```python
from build123d import *

# Parameters (mm, degrees)
F0_R         = 0.875
F1_DEPTH     = 12
F2_R         = 1.75
F3_DEPTH     = 4.001
F4_DEPTH     = 2
F5_T4_DEPTH  = 12
F5_T10_DEPTH = 12
F5_T16_DEPTH = 12
F5_T23_DEPTH = 12
F5_T29_DEPTH = 12
F5_T35_DEPTH = 12
F5_T41_DEPTH = 12
F5_T47_DEPTH = 12
F5_T54_DEPTH = 12
F5_T60_DEPTH = 12
F5_T63_DEPTH = 14.2867319519
F5_T65_DEPTH = 22.2867319519
F6_R         = 1


# Not quite as in the source:
# - a fillet or chamfer that OpenCascade refuses, or shapes differently, is made with other operations: its cross-section is extruded or revolved along the edge and cut away or added


with BuildPart() as f1:
    # F0 (on Top) → F1 (new body)
    with BuildSketch(Plane.XY):
        Polygon((16.5, -5.25), (11.625, -5.25), (-11.625, -5.25), (-16.5, -5.25), (-16.5, -7.25), (16.5, -7.25), align=None)
        Polygon((-11.625, -5.25), (-11.625, 7.25), (-16.5, 7.25), (-16.5, -3.25), (-16.5, -5.25), align=None)
        with Locations((-13.5, 1)):
            Circle(F0_R, mode=Mode.SUBTRACT)
        Polygon((16.5, -3.25), (16.5, 7.25), (11.625, 7.25), (11.625, -5.25), (16.5, -5.25), align=None)
        with Locations((13.5, 1)):
            Circle(F0_R, mode=Mode.SUBTRACT)
        Polygon((25.5, -3.25), (16.5, -3.25), (16.5, -5.25), (16.5, -7.25), (25.5, -7.25), align=None)
        Polygon((-16.5, -5.25), (-16.5, -3.25), (-25.5, -3.25), (-25.5, -7.25), (-16.5, -7.25), align=None)
    extrude(amount=F1_DEPTH)

    # F2 (on face) → F3 (cut, through all)
    with BuildSketch(Plane(origin=(0, -3.25, 0), x_dir=(-1, 0, 0), z_dir=(0, 1, 0))):
        with Locations((-21, 6)):
            Circle(F2_R)
        with Locations((21, 6)):
            Circle(F2_R)
    extrude(amount=-F3_DEPTH, mode=Mode.SUBTRACT)

    # F2 (on face) → F4 (cut)
    with BuildSketch(Plane(origin=(0, -3.25, 0), x_dir=(-1, 0, 0), z_dir=(0, 1, 0))):
        Polygon((-18.25, 4.4122867597), (-18.25, 7.5877132403), (-21, 9.1754264805), (-23.75, 7.5877132403), (-23.75, 4.4122867597), (-21, 2.8245735195), align=None)
        with Locations((-21, 6)):
            Circle(F2_R, mode=Mode.SUBTRACT)
        Polygon((21, 9.1754264805), (18.25, 7.5877132403), (18.25, 4.4122867597), (21, 2.8245735195), (23.75, 4.4122867597), (23.75, 7.5877132403), align=None)
        with Locations((21, 6)):
            Circle(F2_R, mode=Mode.SUBTRACT)
    extrude(amount=-F4_DEPTH, mode=Mode.SUBTRACT)

    # F5: chamfer of 2 on 8 edges, made by hand


with BuildPart() as f5_tool2:
    # F5_s3 → F5_t4 (new body)
    with BuildSketch(Plane.XY):
        Polygon((18.5, -3.25), (16.5, -1.25), (16.5, -3.25), align=None)
    extrude(amount=F5_T4_DEPTH)

    split(bisect_by=Plane.YZ.offset(18.25), keep=Keep.TOP)

    split(bisect_by=Plane(origin=(6.4730762114, 0, 11.2116968793), x_dir=(0, 1, 0), z_dir=(-0.5, 0, -0.8660254038)), keep=Keep.TOP)


with BuildPart() as f1_1:
    add(f1.part)

    # F5_t1: union F5_tool2
    add(f5_tool2.part)


with BuildPart() as f5_tool8:
    # F5_s9 → F5_t10 (new body)
    with BuildSketch(Plane.XY):
        Polygon((18.5, -3.25), (16.5, -1.25), (16.5, -3.25), align=None)
    extrude(amount=F5_T10_DEPTH)

    split(bisect_by=Plane.YZ.offset(18.25), keep=Keep.BOTTOM)

    split(bisect_by=Plane(origin=(6.4730762114, 0, 11.2116968793), x_dir=(0, 1, 0), z_dir=(-0.5, 0, -0.8660254038)), keep=Keep.TOP)


with BuildPart() as f1_2:
    add(f1_1.part)

    # F5_t7: union F5_tool8
    add(f5_tool8.part)


with BuildPart() as f5_tool14:
    # F5_s15 → F5_t16 (new body)
    with BuildSketch(Plane.XY):
        Polygon((18.5, -3.25), (16.5, -1.25), (16.5, -3.25), align=None)
    extrude(amount=F5_T16_DEPTH)

    split(bisect_by=Plane(origin=(1.2769237886, 0, -2.2116968793), x_dir=(0, 1, 0), z_dir=(0.5, 0, -0.8660254038)), keep=Keep.TOP)

    split(bisect_by=Plane.YZ.offset(18.25), keep=Keep.BOTTOM)

    split(bisect_by=Plane(origin=(6.4730762114, 0, 11.2116968793), x_dir=(0, 1, 0), z_dir=(0.5, 0, 0.8660254038)), keep=Keep.TOP)


with BuildPart() as f1_3:
    add(f1_2.part)

    # F5_t13: union F5_tool14
    add(f5_tool14.part)


with BuildPart() as f5_tool21:
    # F5_s22 → F5_t23 (new body)
    with BuildSketch(Plane.XY):
        Polygon((18.5, -3.25), (16.5, -1.25), (16.5, -3.25), align=None)
    extrude(amount=F5_T23_DEPTH)

    split(bisect_by=Plane(origin=(1.2769237886, 0, -2.2116968793), x_dir=(0, 1, 0), z_dir=(-0.5, 0, 0.8660254038)), keep=Keep.TOP)

    split(bisect_by=Plane.YZ.offset(18.25), keep=Keep.TOP)


with BuildPart() as f1_4:
    add(f1_3.part)

    # F5_t20: union F5_tool21
    add(f5_tool21.part)


with BuildPart() as f5_tool27:
    # F5_s28 → F5_t29 (new body)
    with BuildSketch(Plane.XY):
        Polygon((18.5, -3.25), (16.5, -1.25), (16.5, -3.25), align=None)
    extrude(amount=F5_T29_DEPTH)

    split(bisect_by=Plane(origin=(1.2769237886, 0, -2.2116968793), x_dir=(0, 1, 0), z_dir=(-0.5, 0, 0.8660254038)), keep=Keep.TOP)

    split(bisect_by=Plane.YZ.offset(18.25), keep=Keep.BOTTOM)


with BuildPart() as f1_5:
    add(f1_4.part)

    # F5_t26: union F5_tool27
    add(f5_tool27.part)


with BuildPart() as f5_tool33:
    # F5_s34 → F5_t35 (new body)
    with BuildSketch(Plane.XY):
        Polygon((-16.5, -1.25), (-18.5, -3.25), (-16.5, -3.25), align=None)
    extrude(amount=F5_T35_DEPTH)

    split(bisect_by=Plane(origin=(-6.4730762114, 0, 11.2116968793), x_dir=(0, 1, 0), z_dir=(0.5, 0, -0.8660254038)), keep=Keep.TOP)

    split(bisect_by=Plane.YZ.offset(-18.25), keep=Keep.TOP)


with BuildPart() as f1_6:
    add(f1_5.part)

    # F5_t32: union F5_tool33
    add(f5_tool33.part)


with BuildPart() as f5_tool39:
    # F5_s40 → F5_t41 (new body)
    with BuildSketch(Plane.XY):
        Polygon((-16.5, -1.25), (-18.5, -3.25), (-16.5, -3.25), align=None)
    extrude(amount=F5_T41_DEPTH)

    split(bisect_by=Plane(origin=(-6.4730762114, 0, 11.2116968793), x_dir=(0, 1, 0), z_dir=(0.5, 0, -0.8660254038)), keep=Keep.TOP)

    split(bisect_by=Plane.YZ.offset(-18.25), keep=Keep.BOTTOM)


with BuildPart() as f1_7:
    add(f1_6.part)

    # F5_t38: union F5_tool39
    add(f5_tool39.part)


with BuildPart() as f5_tool45:
    # F5_s46 → F5_t47 (new body)
    with BuildSketch(Plane.XY):
        Polygon((-16.5, -1.25), (-18.5, -3.25), (-16.5, -3.25), align=None)
    extrude(amount=F5_T47_DEPTH)

    split(bisect_by=Plane(origin=(-6.4730762114, 0, 11.2116968793), x_dir=(0, 1, 0), z_dir=(-0.5, 0, 0.8660254038)), keep=Keep.TOP)

    split(bisect_by=Plane.YZ.offset(-18.25), keep=Keep.TOP)

    split(bisect_by=Plane(origin=(-1.2769237886, 0, -2.2116968793), x_dir=(0, 1, 0), z_dir=(-0.5, 0, -0.8660254038)), keep=Keep.TOP)


with BuildPart() as f1_8:
    add(f1_7.part)

    # F5_t44: union F5_tool45
    add(f5_tool45.part)


with BuildPart() as f5_tool52:
    # F5_s53 → F5_t54 (new body)
    with BuildSketch(Plane.XY):
        Polygon((-16.5, -1.25), (-18.5, -3.25), (-16.5, -3.25), align=None)
    extrude(amount=F5_T54_DEPTH)

    split(bisect_by=Plane.YZ.offset(-18.25), keep=Keep.TOP)

    split(bisect_by=Plane(origin=(-1.2769237886, 0, -2.2116968793), x_dir=(0, 1, 0), z_dir=(0.5, 0, 0.8660254038)), keep=Keep.TOP)


with BuildPart() as f1_9:
    add(f1_8.part)

    # F5_t51: union F5_tool52
    add(f5_tool52.part)


with BuildPart() as f5_tool58:
    # F5_s59 → F5_t60 (new body)
    with BuildSketch(Plane.XY):
        Polygon((-16.5, -1.25), (-18.5, -3.25), (-16.5, -3.25), align=None)
    extrude(amount=F5_T60_DEPTH)

    split(bisect_by=Plane.YZ.offset(-18.25), keep=Keep.BOTTOM)

    split(bisect_by=Plane(origin=(-1.2769237886, 0, -2.2116968793), x_dir=(0, 1, 0), z_dir=(0.5, 0, 0.8660254038)), keep=Keep.TOP)


with BuildPart() as f1_10:
    add(f1_9.part)

    # F5_t57: union F5_tool58
    add(f5_tool58.part)

    # F5_s64 → F5_t63 (cut)
    with BuildSketch(Plane.XZ.offset(-1.8933659759)):
        Polygon((25.5, 2), (23.5, 0), (25.5, 0), align=None)
        Polygon((23.5, 12), (25.5, 10), (25.5, 12), align=None)
        Polygon((-25.5, 2), (-23.5, 0), (-25.5, 0), align=None)
        Polygon((-23.5, 12), (-25.5, 10), (-25.5, 12), align=None)
    extrude(amount=F5_T63_DEPTH, mode=Mode.SUBTRACT)

    # F5_s66 → F5_t65 (cut)
    with BuildSketch(Plane.XY.offset(-5.1433659759)):
        Polygon((14.5, 7.25), (16.5, 5.25), (16.5, 7.25), align=None)
        Polygon((-16.5, 5.25), (-14.5, 7.25), (-16.5, 7.25), align=None)
    extrude(amount=F5_T65_DEPTH, mode=Mode.SUBTRACT)

    # F6
    f6_edges = [f1_10.edges().sort_by_distance(p)[0] for p in [
        (-11.625, 7.25, 6),
        (11.625, 7.25, 6),
        (11.625, -5.25, 6),
        (-11.625, -5.25, 6),
    ]]
    fillet(f6_edges, radius=F6_R)


solid = f1_10.part
```
Work out the finished part from the listing and answer in its coordinate system (mm). A direction names the side the tool comes from. Round coordinates to 2 decimals unless told otherwise and drop trailing zeros. Write each loop counter-clockwise with the first axis right and the second up, starting at its lowest first coordinate (ties: lowest second). Pieces come first, ordered by that corner, then holes. Notation, with made-up numbers: (-1, 59.5) -> (48, 59.5) arc R30 ccw to (48, 87.5) -> close; hole circle Ø8 at (31, 44). An arc over 180 degrees is marked (long way). Write each question's results on one line, items separated by ' | '.
Q1. Section D-D, the plane y = 1 is taken. Write down the section's boundary in (x, z) (3 decimals), then the cut area to 3 significant figures.
Data:
outline: (-16.5, 0) -> (-14.375, 0) -> (-14.375, 12) -> (-16.5, 12) -> close; (-12.625, 0) -> (-11.625, 0) -> (-11.625, 12) -> (-12.625, 12) -> close; (11.625, 0) -> (12.625, 0) -> (12.625, 12) -> (11.625, 12) -> close; (14.375, 0) -> (16.5, 0) -> (16.5, 12) -> (14.375, 12) -> close | area: 75.0 mm^2
Q2. Flat-ended cylindrical pins translate along their axes: P1, Ø3, axis at x = 20, z = 6.5, coming from the +Y side; P2, Ø5, axis at y = 2, z = 3, coming from the +X side; P3, Ø3.5, axis at x = 22, z = 3.5, coming from the +Y side. Find the tip coordinate at first contact, or state that the pin passes through.
Data:
P1: y = -5.25 | P2: x = 16.5 | P3: y = -3.25
Q3. Section A-A, the plane y = -3.75 is taken. Write down the section's boundary in (x, z) (3 decimals), then the cut area to 3 significant figures.
Data:
outline: (-25.5, 2) -> (-23.5, 0) -> (-11.625, 0) -> (-11.625, 12) -> (-23.5, 12) -> (-25.5, 10) -> close; (11.625, 0) -> (23.5, 0) -> (25.5, 2) -> (25.5, 10) -> (23.5, 12) -> (11.625, 12) -> close; hole (-23.75, 4.412) -> (-21, 2.825) -> (-18.25, 4.412) -> (-18.25, 7.588) -> (-21, 9.175) -> (-23.75, 7.588) -> close; hole (18.25, 4.412) -> (21, 2.825) -> (23.75, 4.412) -> (23.75, 7.588) -> (21, 9.175) -> (18.25, 7.588) -> close | area: 273 mm^2
Q4. Section C-C, the plane y = -1.75 is taken. Write down the section's boundary in (x, z) (3 decimals), then the cut area to 3 significant figures.
Data:
outline: (-17, 0) -> (-11.625, 0) -> (-11.625, 12) -> (-17, 12) -> close; (11.625, 0) -> (17, 0) -> (17, 12) -> (11.625, 12) -> close | area: 129 mm^2
Q5. Section B-B, the plane z = 1 is taken. Write down the section's boundary in (x, y) (3 decimals).
Data:
outline: (-24.5, -7.25) -> (24.5, -7.25) -> (24.5, -3.25) -> (18.5, -3.25) -> (16.5, -1.25) -> (16.5, 5.25) -> (14.5, 7.25) -> (12.625, 7.25) arc R1 ccw to (11.625, 6.25) -> (11.625, -4.25) arc R1 cw to (10.625, -5.25) -> (-10.625, -5.25) arc R1 cw to (-11.625, -4.25) -> (-11.625, 6.25) arc R1 ccw to (-12.625, 7.25) -> (-14.5, 7.25) -> (-16.5, 5.25) -> (-16.5, -1.25) -> (-18.5, -3.25) -> (-24.5, -3.25) -> close; hole circle Ø1.75 at (-13.5, 1); hole circle Ø1.75 at (13.5, 1)
Q6. Which of the six approach directions +Z, -Z, +X, -X, +Y, -Y give full straight-line access (tool end or side, diameter ignored) to faces 4 (the flat face through (-24, -3.25, 6)), 5 (the cylindrical face through (-11.926, 6.965, 6.084)), 6 (the flat face through (15.49, 6.26, 5.92)), 7 (the flat face through (24.5, -5.2, 1)), 8 (the flat face through (-22.36, -4.24, 3.61))?
Data:
face 4: +Z, -Z, -X, +Y | face 5: +Z, -Z, +Y | face 6: +Z, -Z, +X, +Y | face 7: -Z, +X, +Y, -Y | face 8: +Y
Q7. Determine the mould class of faces 1 (the cylindrical face through (12.626, 1.038, 5.916)), 2 (the flat face through (-24.5, -5.2, 11)), 3 (the flat face through (-18.25, -4, 6)) for opening direction Z: released by +Z, released by -Z, zero draft, split by the parting line, or undercut.
Data:
face 1: zero draft | face 2: released by +Z | face 3: undercut
Q8. Straight lines are drawn through the part: line 1 along X through (y, z) = (-4, 6) (3 decimals); line 2 along X through (y, z) = (1.5, 10.5) (3 decimals); line 3 along X through (y, z) = (2.5, 6.25) (3 decimals). For each, find the intervals that lie inside material, in ascending order. Write a range as [from, to].
Data:
line 1: [-25.5, -23.75], [-18.25, -11.625], [11.625, 18.25], [23.75, 25.5] | line 2: [-16.5, -14.218], [-12.782, -11.625], [11.625, 12.782], [14.218, 16.5] | line 3: [-16.5, -11.625], [11.625, 16.5]
